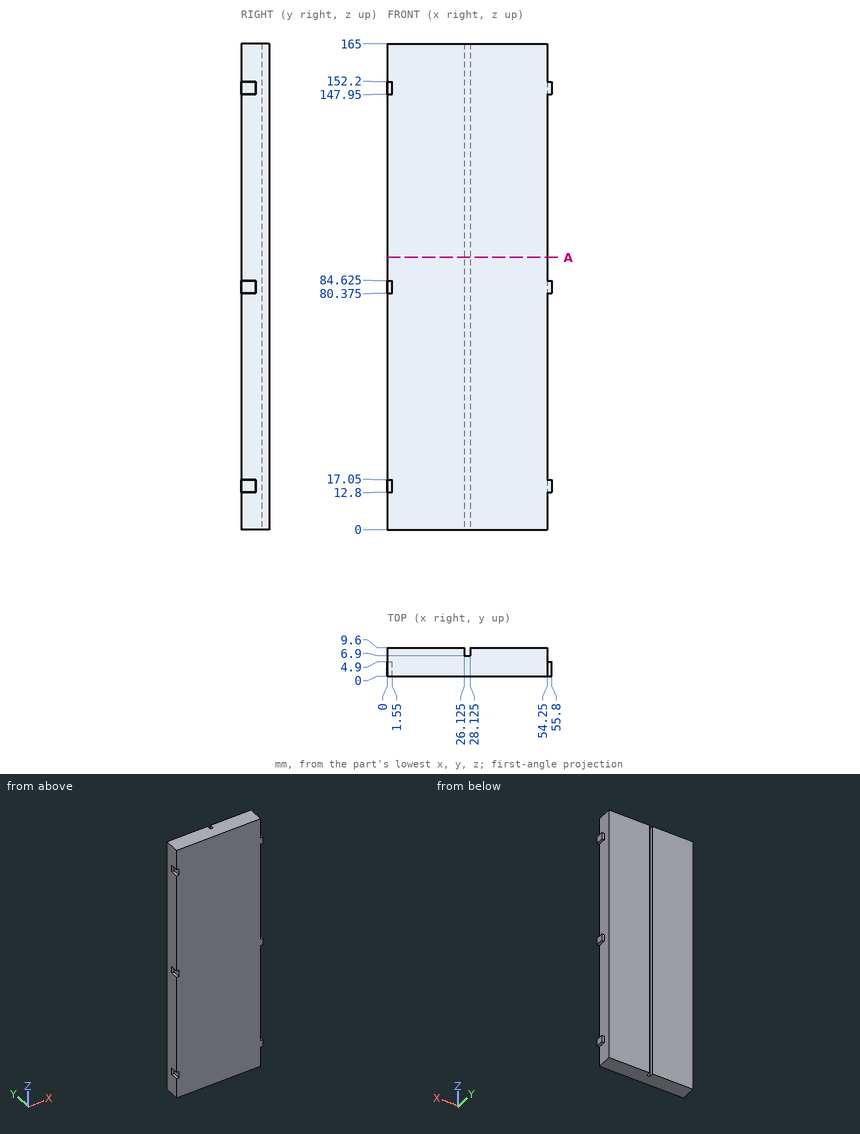
Design review of the part shown in the three views and the two pictorial views. Dimensions are in mm from the part's minimum x, y and z. Coordinates: 2 decimals unless noted, no trailing zeros. Order: outer loops, then holes, each group sorted by start corner. A loop starts at its lowest first (then second) coordinate and runs counter-clockwise, first axis right, second up.
1) Clearance check with flat-ended pins moving along their axes: pin 1 (5 mm diameter, centred on y = 7, z = 61, fed in from +X); pin 2 (0.5 mm diameter, centred on x = 55.5, y = 3.5, fed in from -Z); pin 3 (1 mm diameter, centred on x = 27, z = 84, fed in from +Y). State where each tip first meets the part, or that it passes through.
2) Wall thickness on line 1 along X through (y, z) = (7, 29) (3 decimals); line 2 along X through (y, z) = (3.75, 17); line 3 along X through (y, z) = (4.75, 140.5): over which ranges is each line inside the solid? List them lowest first.
3) Take a section at A-A, the plane z = 92.5. Give the boundary of the cut face in (x, y) (3 decimals), and give its area (3 significant figures).
Returned:
1. pin 1: stops at x = 54.25
1. pin 2: stops at z = 12.8
1. pin 3: stops at y = 6.9
2. line 1: x = 0 to 26.125, 28.125 to 54.25
2. line 2: x = 1.55 to 55.8
2. line 3: x = 0 to 54.25
3. outline: (0, 0) - (54.25, 0) - (54.25, 9.6) - (28.125, 9.6) - (28.125, 6.9) - (26.125, 6.9) - (26.125, 9.6) - (0, 9.6) - close
3. area: 515 mm2
